Build history of the part. All positions in model axes, mm. A direction names the side the tool comes from. Round coordinates to 2 decimals unless told otherwise and drop trailing zeros. Order: outer loops, then holes, each group sorted by start corner. A loop starts at its lowest first (then second) coordinate and runs counter-clockwise, first axis right, second up. Notation, with made-up numbers: (65, 24) -> (103, 24) arc R19 ccw to (103, 35) -> close; hole circle Ø10 at (20, 64.5). An arc over 180 degrees is marked (long way). Use a Markdown table: item, result. Add a question column.
Item 1: Slice it at D-D, the plane y = 4.25. Give the cut face in (x, z).
Item 2: Two-plate mould, pull along Y, no slides. Class faces 4 (the face through (-10, -2, 8)), 5 (the face through (-1.45, 3.07, 16.56)), 6 (the face through (9, 10, 8)): released by +Y, released by -Y, zero draft, split by the parting line, or undercut.
Item 3: 3-axis set-ups, long thin cutter, end or side, ignore diameter. For faces 1 (the face through (-10, -1, 10)), 2 (the face through (3.869, 6.979, 4.034)), 3 (the face through (-0.52, 3.4, 18.95)): which of +Z, -Z, +X, -X, +Y, -Y reach the whole face in a straight line?
Item 4: Probe L1, parallel to Z at x = 0, y = 2.5; L2, parallel to Z at x = -6.5, y = 8.5; L3, parallel to Z at x = 0, y = 8.55 (3 decimals). List the from-to ranges inside material, lowest first.
Item 5: Pin check, flat tips, straight feed: pin 1 (10 mm diameter, centred on x = -3, z = 13, fed in from +Y); pin 2 (9 mm diameter, centred on x = 0, z = 7, fed in from +Y); pin 3 (0.6 mm diameter, centred on x = 9.5, y = -0.5, fed in from +Z); pin 4 (10.5 mm diameter, centred on x = 0, z = 5.5, fed in from +Y). Stop position of each tip, or through.
Item 6: Slice it at B-B, the plane y = 2. Give the cut face in (x, z), plus the area to 3 significant figures.
Item 7: Slice it at A-A, the plane y = 8. State how many separate pieces and enclosed holes the cut face has, plus the area to 3 significant figures.
from build123d import *

# Parameters (mm, degrees)
F0_W            = 30
F0_H            = 10
F1_DEPTH        = 30
F6_DEPTH        = 25
F7_R            = 8
F8_W            = 30
F8_H            = 6
F9_DEPTH        = 2
F11_D           = 5.5
F11_DEPTH       = 100
F11_CBORE_D     = 9.75
F11_CBORE_DEPTH = 5
F11_TIP         = 1.6523667023
F12_R           = 2.75
F13_DEPTH       = 2
F14_SIZE2       = 1.7320508076
F14_SIZE        = 1
F14_2_SIZE2     = 1.7320508076
F14_2_SIZE      = 1


with BuildPart() as f1:
    # F0 (on Top) → F1 (new body)
    with BuildSketch(Plane.XY):
        with Locations((0, 5)):
            Rectangle(F0_W, F0_H)
    extrude(amount=F1_DEPTH)

    # F3 (on offset) → F4 (revolve, cut)
    with BuildSketch(Plane.XZ.offset(-12)):
        Polygon((16.9375651661, 30.751099481), (11.3471165957, 34.963804643), (-15.5656658205, -0.7506638978), (-9.9752172501, -4.9633690599), align=None)
        Polygon((9.7408888818, 14.3880629064), (7.7443001067, 15.8926004643), (4.7352249909, 11.8994229141), (6.7318137661, 10.3948853562), align=None)
    revolve(axis=Axis((-2.1092746124, 12, 17.1065703726), (-0.6018150232, 0, -0.79863551)), mode=Mode.SUBTRACT)

    # F5 (on offset) → F6 (intersect)
    with BuildSketch(Plane.XZ.offset(-12)):
        Polygon((3.6727298394, -14.6139401428), (23.5988721657, 11.0938824045), (-9.6680302551, 36.8790702076), (-29.5941725814, 11.1712476603), align=None)
    extrude(amount=F6_DEPTH, mode=Mode.INTERSECT)

    # F7
    f7_edges = [f1.edges().sort_by_distance(p)[0] for p in [
        (-15, 5, 30),
        (15, 5, 17.758871),
    ]]
    fillet(f7_edges, radius=F7_R)

    # F8 (on face) → F9 (join)
    with BuildSketch(Plane.XZ):
        with Locations((0, 7)):
            Rectangle(F8_W, F8_H)
    extrude(amount=F9_DEPTH)

    # F11
    with Locations(Plane(origin=(0, 10, 0), x_dir=(-1, 0, 0), z_dir=(0, 1, 0))):
        with Locations((0, 7)):
            CounterBoreHole(F11_D / 2, F11_CBORE_D / 2, F11_CBORE_DEPTH, depth=F11_DEPTH)
            with Locations((0, 0, -(F11_DEPTH + F11_TIP / 2))):  # 118° drill point
                Cone(0, F11_D / 2, F11_TIP, mode=Mode.SUBTRACT)

    # F12 (on face) → F13 (cut)
    with BuildSketch(Plane.XZ.offset(2)):
        with BuildLine():
            ThreePointArc((5.5302698775, 4), (6.0982775835, 5.4524550305), (6.2915725314, 7))
            ThreePointArc((6.2915725314, 7), (6.0982775835, 8.5475449695), (5.5302698775, 10))
            Line((5.5302698775, 10), (-5.5302698775, 10))
            ThreePointArc((-5.5302698775, 10), (-6.2915725314, 7), (-5.5302698775, 4))
            Line((-5.5302698775, 4), (5.5302698775, 4))
        make_face()
        with Locations((0, 7)):
            Circle(F12_R, mode=Mode.SUBTRACT)
    extrude(amount=-F13_DEPTH, mode=Mode.SUBTRACT)

    # F14
    f14_edges = [f1.edges().sort_by_distance(p)[0] for p in [
        (10.265135, -2, 4),
    ]]
    f14_side = f1.faces().sort_by_distance((10.51932, -2, 7))[0]
    chamfer(f14_edges, length=F14_SIZE, length2=F14_SIZE2, reference=f14_side)

    # F14#2
    f14_2_edges = [f1.edges().sort_by_distance(p)[0] for p in [
        (-10.265135, -2, 4),
    ]]
    f14_2_side = f1.faces().sort_by_distance((-10.51932, -2, 7))[0]
    chamfer(f14_2_edges, length=F14_2_SIZE, length2=F14_2_SIZE2, reference=f14_2_side)


solid = f1.part
Check sheet entries:
| question | item | result |
|---|---|---|
| 1 | outline | (-15, 0) -> (15, 0) -> (15, 13.84) arc R8 ccw to (11.9, 20.16) -> (-0.79, 30) -> (-7, 30) arc R8 ccw to (-15, 22) -> close; hole (-8.48, 21.86) -> (-5.11, 19.32) -> (-2.1, 23.31) -> (-5.47, 25.85) -> close; hole circle Ø5.5 at (0, 7); hole (0.84, 14.83) -> (4.21, 12.29) -> (7.22, 16.29) -> (3.85, 18.82) -> close |
| 2 | face 4 | released by -Y |
| 2 | face 5 | undercut |
| 2 | face 6 | released by +Y |
| 3 | face 1 | +Z, +X, -X, -Y |
| 3 | face 2 | +Y |
| 3 | face 3 | none |
| 4 | L1 | 0 to 4.25, 9.75 to 15.47, 21.73 to 29.39 |
| 4 | L2 | 0 to 1.21, 21.35 to 24.33, 26.63 to 30 |
| 4 | L3 | 0 to 2.125 |
| 5 | pin 1 | y = 9.3 |
| 5 | pin 2 | y = 5 |
| 5 | pin 3 | z = 10 |
| 5 | pin 4 | y = 10 |
| 6 | outline | (-15, 0) -> (15, 0) -> (15, 13.84) arc R8 ccw to (11.9, 20.16) -> (-0.79, 30) -> (-7, 30) arc R8 ccw to (-15, 22) -> close; hole (-5.98, 19.97) -> (1.71, 14.18) -> (4.72, 18.17) -> (-2.97, 23.97) -> close; hole circle Ø5.5 at (0, 7) |
| 6 | area | 715 mm2 |
| 7 | separate pieces | 2 |
| 7 | enclosed holes | 2 |
| 7 | area | 365 mm2 |
